from build123d import *

# Parameters (mm, degrees)
F1_R     = 16
F1_W     = 7
F1_H     = 7
F2_DEPTH = 19
F3_SIZE  = 1
F4_R     = 1
F5_SIZE  = 1
F6_SIZE  = 1


with BuildPart() as f2:
    # F1 (on Top) → F2 (new body)
    with BuildSketch(Plane.XY):
        with BuildLine():
            ThreePointArc((17.1245437895, -7), (18.1528793874, -3.5669272416), (18.5, 0))
            ThreePointArc((18.5, 0), (13.081475452, 13.081475452), (0, 18.5))
            ThreePointArc((0, 18.5), (-15.3582225534, -10.3138256724), (17.1245437895, -7))
        make_face()
        Circle(F1_R, mode=Mode.SUBTRACT)
        with BuildLine():
            ThreePointArc((0, 18.5), (13.081475452, 13.081475452), (18.5, 0))
            Line((18.5, 0), (18.5, 18.5))
            Line((18.5, 18.5), (0, 18.5))
        make_face()
        Polygon((18.5, 18.5), (18.5, 0), (25.5, 0), (25.5, 45), (18.5, 45), align=None)
        with BuildLine():
            Line((18.5, -7), (18.5, 0))
            ThreePointArc((18.5, 0), (18.1528793874, -3.5669272416), (17.1245437895, -7))
            Line((17.1245437895, -7), (18.5, -7))
        make_face()
        with Locations((22, -3.5)):
            Rectangle(F1_W, F1_H)
    extrude(amount=F2_DEPTH)

    # F3
    f3_edges = [f2.edges().sort_by_distance(p)[0] for p in [
        (25.5, -7, 9.5),
    ]]
    chamfer(f3_edges, length=F3_SIZE)

    # F4
    f4_edges = [f2.edges().sort_by_distance(p)[0] for p in [
        (-16, 0, 19),
        (-16, 0, 0),
    ]]
    fillet(f4_edges, radius=F4_R)

    # F5
    f5_edges = [f2.edges().sort_by_distance(p)[0] for p in [
        (9.25, 18.5, 19),
        (-15.358223, -10.313826, 19),
        (-15.358223, -10.313826, 0),
        (9.25, 18.5, 0),
    ]]
    chamfer(f5_edges, length=F5_SIZE)

    # F6
    f6_edges = [f2.edges().sort_by_distance(p)[0] for p in [
        (18.5, 45, 9.5),
        (22, 45, 0),
        (22, 45, 19),
        (25.5, 45, 9.5),
        (18.5, 31.75, 19),
        (18.5, 31.75, 0),
        (20.812272, -7, 19),
        (20.812272, -7, 0),
    ]]
    chamfer(f6_edges, length=F6_SIZE)


solid = f2.part
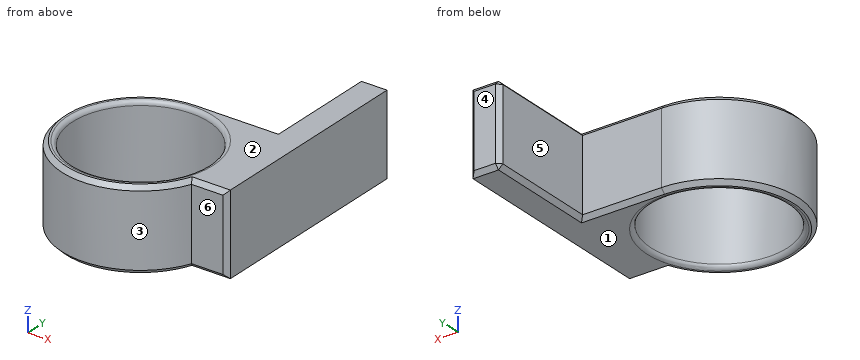
Verification items for the finished model (mm, model axes). Face numbers are marked on the shaded views. A direction names the side the tool comes from. Give positions to 0.01 mm unless a question says otherwise; leave off trailing zeros. Write each loop counter-clockwise with the first axis right and the second up, starting at its lowest first coordinate (ties: lowest second). Pieces come first, ordered by that corner, then holes. Notation, with made-up numbers: M 60,-19 L 102,-19 A18 ccw 102,-14 Z; hole C 89,54.25 d1. An arc over 180 degrees is marked long. Put each result on its own line as item: value. Start each with the question number.
1. Scan lines: line 1 along Y through (x, z) = (0, 12.5); line 2 along Y through (x, z) = (-9, 18); line 3 along X through (y, z) = (10, 2). Record each from-to range of solid material in increasing order. Write a range as [from, to].
2. Draft check along Z on the marked faces 1, 2 and 3. Enter one of: +Z half, -Z half, draft (parallel to the pull), parting line (faces both ways), or undercut.
3. Set-up check for the marked faces 4, 5 and 6: record each of +Z, -Z, +X, -X, +Y, -Y from which the full face is reachable in a straight line by a thin tool's end or side.
4. Go/stop test with flat-tipped pins: pin 1 Ø3 at (x, z) = (-8.5, 9) entering from +Y; pin 2 Ø1 at (x, z) = (5, 5) entering from +Y; pin 3 Ø1.5 at (x, z) = (19, 6.5) entering from -Y. Record where each tip stops, or that it passes through.
5. Section check B-B (z = 13). Record the cut outline in (x, y), and give its area (3 significant figures).
6. Section check C-C (y = 41.5). Record the cut outline in (x, z).
7. Section check A-A (y = 0). Record the cut outline in (x, z).
Answer list:
1. line 1: [-18.5, -16], [16, 18.5]
1. line 2: [-16.16, -13.23], [13.23, 16.16]
1. line 3: [-15.56, -12.49], [12.49, 25.5]
2. face 1: -Z half
2. face 2: +Z half
2. face 3: draft
3. face 4: +Z, -Z, +X, -X, +Y
3. face 5: +Z, -Z, -X, +Y
3. face 6: +Z, -Z, +X, -Y
4. pin 1: y = 17.12
4. pin 2: y = 18.5
4. pin 3: y = -7
5. outline: M 0,18.5 A18.5 ccw long 17.12,-7 L 24.5,-7 L 25.5,-6 L 25.5,44 L 24.5,45 L 19.5,45 L 18.5,44 L 18.5,18.5 Z; hole C 0,0 d32
5. area: 710 mm2
6. outline: M 18.5,1 L 19.5,0 L 25.5,0 L 25.5,19 L 19.5,19 L 18.5,18 Z
7. outline: M -18.5,1 L -17.5,0 L -17,0 A1 ccw -16,1 L -16,18 A1 ccw -17,19 L -17.5,19 L -18.5,18 Z; M 16,1 A1 ccw 17,0 L 25.5,0 L 25.5,19 L 17,19 A1 ccw 16,18 Z
